Here's how the part is built. I have some questions about the finished solid (model axes, mm). A direction names the side the tool comes from. Coordinates: 2 decimals unless noted, no trailing zeros. Write each loop counter-clockwise with the first axis right and the second up, starting at its lowest first coordinate (ties: lowest second). Pieces come first, ordered by that corner, then holes. Notation, with made-up numbers: (41, 54.5) -> (45, 54.5) arc R28 cw to (45, 82.5) -> close; hole circle Ø11 at (38.5, -3.75). An arc over 180 degrees is marked (long way). Put each result on its own line as item: value. Start each with the question number.
Item 1: I want a section at A-A, the plane y = 95. List the corners of the cut face in (x, z) for me.
Item 2: For pin 1 (10 mm diameter, centred on y = 50.5, z = 13, fed in from -X); pin 2 (12 mm diameter, centred on y = 68.5, z = 24.5, fed in from -X); pin 3 (10 mm diameter, centred on x = -19, y = 74.5, fed in from +Z); pin 4 (8 mm diameter, centred on x = 25.5, z = -8, fed in from -Y), each with a flat end and sliding along its axis, tell me the tip position at first contact or that it passes through.
Item 3: If we mould it in two halves opening along X, with no side actions, what happens to faces 4 (the face through (20, 0, -20)), 5 (the face through (-7.21, 54.25, -22.89)), 6 (the face through (-45.856, 2.465, 6.021))? For each: released by +X, released by -X, zero draft, split by the parting line, or undercut.
Item 4: On a 3-axis mill with a long thin cutter (end or side, diameter ignored), from which of +Z, -Z, +X, -X, +Y, -Y can I reach the whole of each face in a straight line? I mean faces 1 (the face through (-8, 107, -23)), 2 (the face through (-31.5, 5, -10.9)), 3 (the face through (-9.131, 11.966, -28.996)). Say none if no direction works.
Item 5: I want a section at B-B, the plane y = 54. List the corners of the cut face in (x, z) for me, then the cut area to 3 significant figures.
Item 6: I need wall thicknesses on line 1 (Z direction, x = 1, y = 39.5); line 2 (X direction, y = 34.5, z = 0); line 3 (X direction, y = 85.5, z = 0). Which ranges of each line are inside material? Lowest first, please. Write a range as [from, to].
from build123d import *

# Parameters (mm, degrees)
SKETCH2_R          = 37.5
CUT_EXTRUDE1_DEPTH = 47


with BuildPart() as part:
    # Sketch1 → Revolve1 (revolve)
    with BuildSketch(Plane.XY, mode=Mode.PRIVATE) as revolve1_sk:
        Polygon((24, 154), (27.5, 154), (27.5, 69.8), (28, 69.3), (28, 25), (32, 25), (33, 24), (33, 14.4), (30.4, 14.4), (30.4, 9.6), (33, 9.6), (33, 5), (46.25, 5), (46.25, 0), (26.775, 0), (26.35, 0.5), (25.925, 0), (24, 0), align=None)
    revolve(revolve1_sk.sketch.rotate(Axis((0, 0, 0), (0, 1, 0)), 90), axis=Axis((0, 0, 0), (0, 1, 0)))

    # Sketch2 → Cut-Extrude1 (cut)
    with BuildSketch(Plane(origin=(0, 154, 0), x_dir=(1, 0, 0), z_dir=(0, 1, 0))):
        Circle(SKETCH2_R)
    extrude(amount=-CUT_EXTRUDE1_DEPTH, mode=Mode.SUBTRACT)


solid = part.part
Calculated:
1. outline: circle Ø55 at (0, 0); hole circle Ø48 at (0, 0)
2. pin 1: stops at x = -26.83
2. pin 2: stops at x = -21.02
2. pin 3: stops at z = 23.67
2. pin 4: stops at y = 0
3. face 4: zero draft
3. face 5: undercut
3. face 6: split by the parting line
4. face 1: +Z, -Z, +X, -X, +Y
4. face 2: +Y
4. face 3: none
5. outline: circle Ø56 at (0, 0); hole circle Ø48 at (0, 0)
5. area: 653 mm2
6. line 1: z = [-27.98, -23.98], [23.98, 27.98]
6. line 2: x = [-28, -24], [24, 28]
6. line 3: x = [-27.5, -24], [24, 27.5]
